Here's how the part is built. I have some questions about the finished solid (model axes, mm). Give positions to 0.01 mm unless a question says otherwise; leave off trailing zeros. Loops run counter-clockwise (first coordinate to the right, second up) from the corner with the lowest first, then second, coordinate; pieces in that order, holes last. Notation, with made-up numbers: M 58,49.25 L 112,49.25 A20 ccw 112,64.25 Z; hole C 66,25 d10. An arc over 180 degrees is marked long. Answer as CSV lines item,"result". Start each with the question number.
Item 1: Will these pins go through, and if not, where does the flat tip stop? P1, Ø3, axis at x = 1, y = -8, coming from the -Z side; P2, Ø2, axis at x = 3, y = -161, coming from the +Z side.
Item 2: I want a section at A-A on z = 7. List the corners of the cut face in (x, y) for me, plus the area to 3 significant figures.
Item 3: If I drill on line 1 along Y through (x, z) = (5, -50.8); line 2 along Y through (x, z) = (2.25, -50); line 3 along Z through (x, y) = (5.75, -209.5), over which ranges is the centre line in solid material (lowest first)? Write a range as from..to.
Item 4: If we mould it in two halves opening along Y, with no side actions, what happens to faces 1 (the flat face through (6.35, -100, -36)), 2 (the flat face through (3.131, -106.338, -0.403)), 3 (the cylindrical face through (3.131, -206.197, -49.241))? For each: released by +Y, released by -Y, zero draft, split by the parting line, or undercut.
Item 5: I want a section at C-C on z = -63.5. List the corners of the cut face in (x, y) for me.
Item 6: I want a section at B-B on x = 2.25. Give the number of separate pieces and of enclosed holes in the cut face, plus the area to 3 significant figures.
Item 7: I want a section at D-D on y = -76.2. List the corners of the cut face in (x, z) for me.
from build123d import *

# Parameters (mm, degrees)
BOSS_EXTRUDE1_DEPTH     = 6.35
F_1_1_DIAMETER_HOLE1_D  = 28.575
F_1_4_CLEARANCE_HOLE1_D = 6.7564
F_1_4_20_TAPPED_HOLE1_D = 5.1054
F_10_24_TAPPED_HOLE1_D  = 3.7973
F_10_CLEARANCE_HOLE1_D  = 5.1054


with BuildPart() as part:
    # Sketch2 → Boss-Extrude1 (new body)
    with BuildSketch(Plane(origin=(0, 0, 0), x_dir=(0, 0, -1), z_dir=(1, 0, 0))):
        with BuildLine():
            Line((68.760512242, -32.839487758), (17.960512242, 17.960512242))
            ThreePointArc((17.960512242, 17.960512242), (-12.514549901, 22.103077632), (-24.641619504, -6.160404876))
            Line((-24.641619504, -6.160404876), (26.158380496, -209.360404876))
            ThreePointArc((26.158380496, -209.360404876), (53.903454898, -228.40969194), (76.2, -203.2))
            Line((76.2, -203.2), (76.2, -50.8))
            ThreePointArc((76.2, -50.8), (74.266540126, -41.079840818), (68.760512242, -32.839487758))
        make_face()
    extrude(amount=BOSS_EXTRUDE1_DEPTH)

    # 1 (1) Diameter Hole1 (through all)
    with Locations(Plane(origin=(6.35, 0, 0), x_dir=(0, 0, -1), z_dir=(1, 0, 0))):
        with Locations((0, 0)):
            Hole(F_1_1_DIAMETER_HOLE1_D / 2)

    # 1/4 Clearance Hole1 (through all)
    with Locations(Plane(origin=(6.35, 0, 0), x_dir=(0, 0, -1), z_dir=(1, 0, 0))):
        with Locations((50.8, -50.8), (50.8, -203.2), (12.320809752, -127.828401175)):
            Hole(F_1_4_CLEARANCE_HOLE1_D / 2)

    # 1/4-20 Tapped Hole1 (through all)
    with Locations(Plane.ZY):
        with Locations((-63.5, -57.7088), (-63.5, -43.8912), (-63.5, -196.2912), (-63.5, -210.1088)):
            Hole(F_1_4_20_TAPPED_HOLE1_D / 2)

    # #10-24 Tapped Hole1 (through all)
    with Locations(Plane.ZY):
        with Locations((-34.925, -50.8), (-11.1125, -50.8)):
            Hole(F_10_24_TAPPED_HOLE1_D / 2)

    # #10 Clearance Hole1 (through all)
    with Locations(Plane.ZY):
        with Locations((-73.025, -76.2), (-73.025, -177.8)):
            Hole(F_10_CLEARANCE_HOLE1_D / 2)


solid = part.part
Result:
1,P1,"z = -45.42"
1,P2,"z = -13.82"
2,outline,"M 0,-76.73 L 6.35,-76.73 L 6.35,-12.46 L 0,-12.46 Z; M 0,12.46 L 6.35,12.46 L 6.35,24.42 L 0,24.42 Z"
2,area,"484 mm^2"
3,line 1,"-228.6..-206.58, -199.82..-54.18, -47.42..-14.88"
3,line 2,"-228.59..-206.48, -199.92..-54.08, -47.52..-14.08"
3,line 3,"-75.41..-65.98, -61.02..-26.19"
4,face 1,"zero draft"
4,face 2,"released by -Y"
4,face 3,"undercut"
5,outline,"M 0,-225.2 L 6.35,-225.2 L 6.35,-212.66 L 0,-212.66 Z; M 0,-207.56 L 6.35,-207.56 L 6.35,-198.84 L 0,-198.84 Z; M 0,-193.74 L 6.35,-193.74 L 6.35,-60.26 L 0,-60.26 Z; M 0,-55.16 L 6.35,-55.16 L 6.35,-46.44 L 0,-46.44 Z; M 0,-41.34 L 6.35,-41.34 L 6.35,-27.58 L 0,-27.58 Z"
6,separate pieces,"1"
6,enclosed holes,"12"
6,area,"16,000 mm^2"
7,outline,"M 0,-76.2 L 6.35,-76.2 L 6.35,-75.58 L 0,-75.58 Z; M 0,-70.47 L 6.35,-70.47 L 6.35,7.13 L 0,7.13 Z"
